Can you work these out from the model? Positions are in its coordinate system, mm. A direction names the side the tool comes from. Give positions to 0.01 mm unless a question says otherwise; leave off trailing zeros. Order: outer loops, then holes, each group sorted by start corner. A loop starts at its lowest first (then second) coordinate and runs counter-clockwise, first axis right, second up. Notation, with made-up numbers: M 43.25,-22 L 92.25,-22 A35 cw 92.25,11 Z; hole C -25,41.25 d1. An arc over 180 degrees is marked long. Answer as a JSON object with one key per item and string values.
```python
from build123d import *

# Parameters (mm, degrees)
EXTRUDE_1_DEPTH     = 3
SKETCH_2_R          = 2.1
CUT_EXTRUDE_1_DEPTH = 3


with BuildPart() as part:
    # 草图1 → 凸台-拉伸1 (new body)
    with BuildSketch(Plane.XY):
        Polygon((-20, 0), (-30, 0), (-30, 40), (70, 40), (70, 0), (60, 0), (40, -20), (40, -30), (0, -30), (0, -20), align=None)
    extrude(amount=EXTRUDE_1_DEPTH)

    # 草图2 → 切除-拉伸1 (cut)
    with BuildSketch(Plane.XY.offset(3)):
        with Locations((10, -7)):
            Circle(SKETCH_2_R)
        with Locations((30, -7)):
            Circle(SKETCH_2_R)
        with Locations((10, -22)):
            Circle(SKETCH_2_R)
        with Locations((30, -22)):
            Circle(SKETCH_2_R)
        with Locations((-20, 10)):
            Circle(SKETCH_2_R)
        with Locations((-20, 32)):
            Circle(SKETCH_2_R)
        with Locations((5, 10)):
            Circle(SKETCH_2_R)
        with Locations((35, 10)):
            Circle(SKETCH_2_R)
        with Locations((60, 10)):
            Circle(SKETCH_2_R)
        with Locations((60, 32)):
            Circle(SKETCH_2_R)
        with Locations((35, 32)):
            Circle(SKETCH_2_R)
        with Locations((5, 32)):
            Circle(SKETCH_2_R)
    extrude(amount=-CUT_EXTRUDE_1_DEPTH, mode=Mode.SUBTRACT)


solid = part.part
```
1) I'm going to push flat-ended pins straight in: pin 1 Ø4 at (x, y) = (5, 10) entering from +Z; pin 2 Ø1.5 at (y, z) = (-24, 2) entering from +X; pin 3 Ø1.5 at (y, z) = (-24.5, 2) entering from -X. Where does each tip first touch, or does it pass through?
Results found:
{"pin 1": "passes through", "pin 2": "stops at x = 40", "pin 3": "stops at x = 0"}
2) For faces 1 (the face through (0, -25, 1)), 2 (the face through (-19.031, 30.137, 1.521)), 3 (the face through (65, 0, 1)), which set-ups out of +Z, -Z, +X, -X, +Y, -Y let a thin tool reach every point of the face, with its end or its side?
Results found:
{"face 1": "+Z, -Z, -X, -Y", "face 2": "+Z, -Z", "face 3": "+Z, -Z, +X, -Y"}
3) I need wall thicknesses on L1, parallel to Y at x = 5, z = 1; L2, parallel to Y at x = 30, z = 0.8; L3, parallel to X at y = 33.5, z = 1.3. Which ranges of each line are inside material? Lowest first, please.
Results found:
{"L1": "y = -30 to 7.9, 12.1 to 29.9, 34.1 to 40", "L2": "y = -30 to -24.1, -19.9 to -9.1, -4.9 to 40", "L3": "x = -30 to -21.47, -18.53 to 3.53, 6.47 to 33.53, 36.47 to 58.53, 61.47 to 70"}
4) I want a section at A-A on y = -7. Write out the boundary of the cut face in (x, z).
Results found:
{"outline": "M -13,0 L 7.9,0 L 7.9,3 L -13,3 Z; M 12.1,0 L 27.9,0 L 27.9,3 L 12.1,3 Z; M 32.1,0 L 53,0 L 53,3 L 32.1,3 Z"}
5) I want a section at C-C on x = 30. Write out the boundary of the cut face in (y, z), and give its area (3 significant figures).
Results found:
{"outline": "M -30,0 L -24.1,0 L -24.1,3 L -30,3 Z; M -19.9,0 L -9.1,0 L -9.1,3 L -19.9,3 Z; M -4.9,0 L 40,0 L 40,3 L -4.9,3 Z", "area": "185 mm²"}
6) I want a section at D-D on y = 32. Write out the boundary of the cut face in (x, z), and give its area (3 significant figures).
Results found:
{"outline": "M -30,0 L -22.1,0 L -22.1,3 L -30,3 Z; M -17.9,0 L 2.9,0 L 2.9,3 L -17.9,3 Z; M 7.1,0 L 32.9,0 L 32.9,3 L 7.1,3 Z; M 37.1,0 L 57.9,0 L 57.9,3 L 37.1,3 Z; M 62.1,0 L 70,0 L 70,3 L 62.1,3 Z", "area": "250 mm²"}
7) Thinking about a two-plate mould opening in Y: for faces 4 (the face through (19, 40, 1)), 5 (the face through (27.9, -6.91, 1.52)), 6 (the face through (20, -30, 1)), which applies, pulls with the +Y half, pulls with the -Y half, needs draft (parallel to the pull), parting line crosses it, or undercut?
Results found:
{"face 4": "pulls with the +Y half", "face 5": "undercut", "face 6": "pulls with the -Y half"}
8) I want a section at B-B on z = 2.45. Count the separate pieces of the cut face and the enclosed holes in it, and give its area (3 significant figures).
Results found:
{"separate pieces": "1", "enclosed holes": "12", "area": "5,430 mm²"}
